```python
from build123d import *

# Parameters (mm, degrees)
IZIM1_R                     = 7
Y_KSEKLIK_EKSTR_ZYON1_DEPTH = 14
Y_KSEKLIK_EKSTR_ZYON3_START = -3
IZIM5_R                     = 8
Y_KSEKLIK_EKSTR_ZYON3_DEPTH = 10
RADYUS1_R                   = 5
L_O_ALTMA1_COUNT            = 2
L_O_ALTMA1_PITCH            = 42


with BuildPart() as part:
    # Çizim1 → Yükseklik-Ekstrüzyon1 (new body)
    with BuildSketch(Plane(origin=(0, 0, 0), x_dir=(1, 0, 0), z_dir=(0, 1, 0))):
        with BuildLine():
            Line((-135.225806452, 45.403225806), (-13.225806452, 45.403225806))
            ThreePointArc((-13.225806452, 45.403225806), (-9.690272546, 43.938759712), (-8.225806452, 40.403225806))
            Line((-8.225806452, 40.403225806), (-8.225806452, -7.596774194))
            ThreePointArc((-8.225806452, -7.596774194), (-9.690272546, -11.132308099), (-13.225806452, -12.596774194))
            Line((-13.225806452, -12.596774194), (-135.225806452, -12.596774194))
            ThreePointArc((-135.225806452, -12.596774194), (-138.761340358, -11.132308099), (-140.225806452, -7.596774194))
            Line((-140.225806452, -7.596774194), (-140.225806452, 40.403225806))
            ThreePointArc((-140.225806452, 40.403225806), (-138.761340358, 43.938759712), (-135.225806452, 45.403225806))
        make_face()
        with Locations(Location((-124.225806452, 16.403225806, 0), (0, 0, 270))):
            Circle(IZIM1_R, mode=Mode.SUBTRACT)
        with Locations(Location((-24.225806452, 16.403225806, 0), (0, 0, 270))):
            Circle(IZIM1_R, mode=Mode.SUBTRACT)
    extrude(amount=Y_KSEKLIK_EKSTR_ZYON1_DEPTH)

    # Çizim5 → Yükseklik-Ekstrüzyon3 (add)
    with BuildSketch(Plane.XY.offset(12.596774194).offset(Y_KSEKLIK_EKSTR_ZYON3_START)):
        with BuildLine():
            ThreePointArc((-55.536681856, 61.121560352), (-74.068812399, 73.999383812), (-92.800827063, 61.414081823))
            Line((-92.800827063, 61.414081823), (-111.725806452, 14))
            Line((-111.725806452, 14), (-36.725806452, 14))
            Line((-36.725806452, 14), (-55.536681856, 61.121560352))
        make_face()
        with Locations((-74.225806452, 54)):
            Circle(IZIM5_R, mode=Mode.SUBTRACT)
    y_kseklik_ekstr_zyon3 = extrude(amount=-Y_KSEKLIK_EKSTR_ZYON3_DEPTH)

    # Radyus1
    radyus1_edges = [part.edges().sort_by_distance(p)[0] for p in [
        (-36.725806452, 14, 4.596774194),
        (-111.725806452, 14, 4.596774194),
    ]]
    fillet(radyus1_edges, radius=RADYUS1_R)

    # LÇoğaltma1: Yükseklik-Ekstrüzyon3 ×2
    with Locations(*[(0, 0, -i * L_O_ALTMA1_PITCH) for i in range(1, L_O_ALTMA1_COUNT)]):
        add(y_kseklik_ekstr_zyon3)


solid = part.part
```
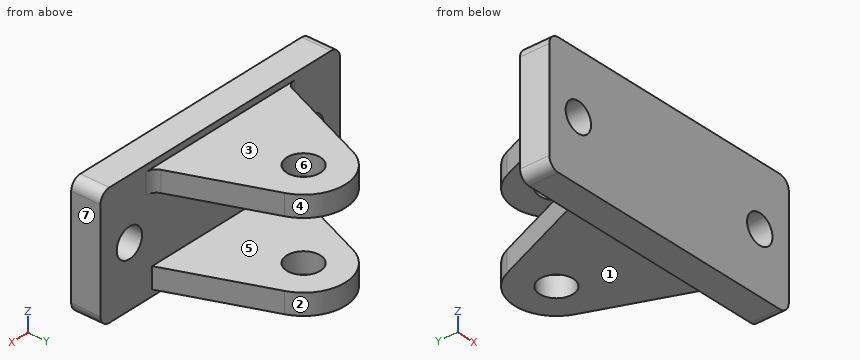
Part model, mm, in its own coordinate system. Face numbers are marked on the shaded views. A direction names the side the tool comes from. Give positions to 0.01 mm unless a question says otherwise; leave off trailing zeros. Order: outer loops, then holes, each group sorted by start corner. A loop starts at its lowest first (then second) coordinate and runs counter-clockwise, first axis right, second up. Notation, with made-up numbers: M -5,23.5 L 17,23.5 A21 cw 17,30.5 Z; hole C 23,21 d7. An arc over 180 degrees is marked long. Use a Markdown table: item, result. Add a question column.
(1) Probe line 1 along Z through (x, y) = (-49.5, 42.5); line 2 along X through (y, z) = (10, -22); line 3 along Y through (x, z) = (-113.5, -3). List the from-to ranges inside material, lowest first. Write a range as [from, to].
(2) Saw through at C-C, the plane x = -122. Give the cut face in (y, z), and give its area (3 significant figures).
(3) Saw through at D-D, the plane y = 54. Give the cut face in (x, z), and give its area (3 significant figures).
(4) 3-axis set-ups, long thin cutter, end or side, ignore diameter. For the marked faces 1, 2 and 3: which of +Z, -Z, +X, -X, +Y, -Y reach the whole face in a straight line?
(5) Drop flat-ended pins along their axis: P1, Ø11, axis at x = -24.23, z = -16.4, coming from the -Y side; P2, Ø4, axis at x = -122.5, z = -9, coming from the +Y side; P3, Ø18, axis at x = -91.5, y = 41, coming from the -Z side; P4, Ø1, axis at x = -114, z = 3, coming from the +Y side. Give the stop position or say it passes through.
(6) Saw through at B-B, the plane y = 18.5. Give the cut face in (x, z), and give its area (3 significant figures).
(7) Mould opens along X. For the marked faces 4, 5, 6 and 7 say: +X half, -X half, draft (parallel to the pull), parting line (faces both ways), or undercut.
(8) Saw through at A-A, the plane z = -35.5. Give the cut face in (x, y).
Answer key:
| question | item | result |
|---|---|---|
| 1 | line 1 | [-42.4, -32.4], [-0.4, 9.6] |
| 1 | line 2 | [-140.23, -128.43], [-120.02, -28.43], [-20.02, -8.23] |
| 1 | line 3 | [0, 14] |
| 2 | outline | M 0,-45.4 L 14,-45.4 L 14,-23.04 L 0,-23.04 Z; M 0,-9.77 L 14,-9.77 L 14,12.6 L 0,12.6 Z |
| 2 | area | 626 mm^2 |
| 3 | outline | M -95.76,-42.4 L -82.23,-42.4 L -82.23,-32.4 L -95.76,-32.4 Z; M -95.76,-0.4 L -82.23,-0.4 L -82.23,9.6 L -95.76,9.6 Z; M -66.23,-42.4 L -52.69,-42.4 L -52.69,-32.4 L -66.23,-32.4 Z; M -66.23,-0.4 L -52.69,-0.4 L -52.69,9.6 L -66.23,9.6 Z |
| 3 | area | 541 mm^2 |
| 4 | face 1 | -Z, +X, -X, +Y |
| 4 | face 2 | +Z, -Z, +Y |
| 4 | face 3 | +Z, +X, -X, +Y |
| 5 | P1 | through |
| 5 | P2 | y = 14 |
| 5 | P3 | z = -42.4 |
| 5 | P4 | y = 14.27 |
| 6 | outline | M -109.93,-42.4 L -38.52,-42.4 L -38.52,-32.4 L -109.93,-32.4 Z; M -109.93,-0.4 L -38.52,-0.4 L -38.52,9.6 L -109.93,9.6 Z |
| 6 | area | 1,430 mm^2 |
| 7 | face 4 | parting line |
| 7 | face 5 | draft |
| 7 | face 6 | undercut |
| 7 | face 7 | +X half |
| 8 | outline | M -140.23,0 L -8.23,0 L -8.23,14 L -36.73,14 L -55.54,61.12 A20 ccw -92.8,61.41 L -111.73,14 L -140.23,14 Z; hole C -74.23,54 d16 |
